from build123d import *

# Parameters (mm, degrees)
SKETCH1_R           = 14.2875
SKETCH1_R_2         = 12.7
BOSS_EXTRUDE1_DEPTH = 1295.4
SKETCH2_R           = 12.7
BOSS_EXTRUDE2_DEPTH = 38.1


with BuildPart() as part:
    # Sketch1 → Boss-Extrude1 (new body)
    with BuildSketch(Plane(origin=(0, 0, 0), x_dir=(1, 0, 0), z_dir=(0, 1, 0))):
        Circle(SKETCH1_R)
        Circle(SKETCH1_R_2, mode=Mode.SUBTRACT)
    extrude(amount=BOSS_EXTRUDE1_DEPTH)

    # Sketch2 → Boss-Extrude2 (add)
    with BuildSketch(Plane.XZ):
        Circle(SKETCH2_R)
        with BuildLine():
            ThreePointArc((-6.985, 9.525), (-8.781051224, 8.781051224), (-9.525, 6.985))
            Line((-9.525, 6.985), (-9.525, -6.985))
            ThreePointArc((-9.525, -6.985), (-8.781051224, -8.781051224), (-6.985, -9.525))
            Line((-6.985, -9.525), (6.985, -9.525))
            ThreePointArc((6.985, -9.525), (8.781051224, -8.781051224), (9.525, -6.985))
            Line((9.525, -6.985), (9.525, 6.985))
            ThreePointArc((9.525, 6.985), (8.781051224, 8.781051224), (6.985, 9.525))
            Line((6.985, 9.525), (-6.985, 9.525))
        make_face(mode=Mode.SUBTRACT)
    extrude(amount=-BOSS_EXTRUDE2_DEPTH)


solid = part.part
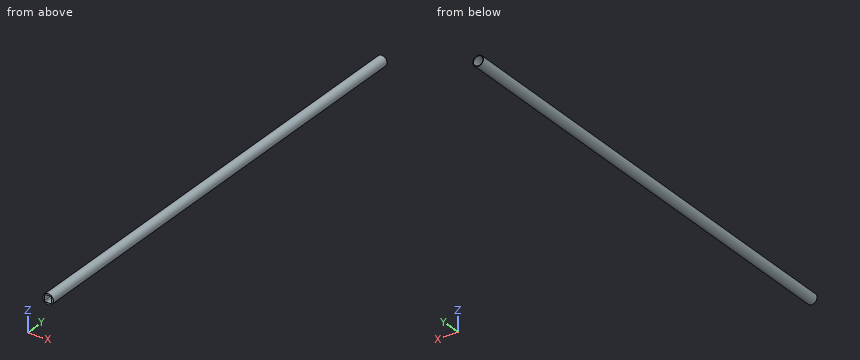
Input: part model. Units: mm. Frame: model coordinates. Give positions to 0.01 mm unless a question says otherwise; leave off trailing zeros. Order: outer loops, then holes, each group sorted by start corner. A loop starts at its lowest first (then second) coordinate and runs counter-clockwise, first axis right, second up. Notation, with made-up numbers: (45.5, 5.5) - (96.5, 5.5) arc R4 ccw to (96.5, 10.5) - close; hole circle Ø2 at (25.5, 89.25). An arc over 180 degrees is marked (long way). Answer as a JSON object with one key per item and string values. Group by question number.
Q1. Cut plane B-B, the plane x = 0. Output: boundary loops of the cut face in (y, z) (1 decimal).
Q2. Cut plane C-C, the plane y = 206. Output: boundary loops of the cut face in (x, z) (1 decimal).
Q3. First-contact query: pin 1 Ø1.5 at (x, y) = (8, 472.5) entering from -Z; pin 2 Ø3 at (x, y) = (-7, 1157) entering from +Z; pin 3 Ø4 at (y, z) = (240.5, 8.5) entering from +X. Flat tips, straight axial feed; report the tip coordinate or a pass-through.
Q4. Cut plane A-A, the plane z = 0. Output: boundary loops of the cut face in (x, y) (1 decimal).
Q5. Line query: probe 1 along X at (y, z) = (433, -2.25); probe 2 along X at (y, z) = (909.5, 0); probe 3 along Y at (x, z) = (3.75, -9.75). Output: solid intervals per line, ascending.
Results:
{
 "1": {"outline": "(0, -14.3) - (1295.4, -14.3) - (1295.4, -12.7) - (38.1, -12.7) - (38.1, -9.5) - (0, -9.5) - close; (0, 9.5) - (38.1, 9.5) - (38.1, 12.7) - (1295.4, 12.7) - (1295.4, 14.3) - (0, 14.3) - close"},
 "2": {"outline": "circle Ø28.6 at (0, 0); hole circle Ø25.4 at (0, 0)"},
 "3": {"pin 1": "z = -12.31", "pin 2": "z = 13.19", "pin 3": "x = 12.72"},
 "4": {"outline": "(-14.3, 0) - (-9.5, 0) - (-9.5, 38.1) - (-12.7, 38.1) - (-12.7, 1295.4) - (-14.3, 1295.4) - close; (9.5, 0) - (14.3, 0) - (14.3, 1295.4) - (12.7, 1295.4) - (12.7, 38.1) - (9.5, 38.1) - close"},
 "5": {"probe 1": "-14.11 to -12.5, 12.5 to 14.11", "probe 2": "-14.29 to -12.7, 12.7 to 14.29", "probe 3": "0 to 38.1"}
}
